CAD build for the part. Positions are in the model's coordinates, mm. Face numbers are marked on the shaded views. A direction names the side the tool comes from. Give positions to 0.01 mm unless a question says otherwise; leave off trailing zeros. Write each loop counter-clockwise with the first axis right and the second up, starting at its lowest first coordinate (ties: lowest second). Pieces come first, ordered by that corner, then holes. Notation, with made-up numbers: (25, 58) - (55, 58) arc R25 ccw to (55, 70) - close; hole circle Ø1 at (56.25, 43.25). An arc over 180 degrees is marked (long way). Answer as a JSON object with one key per item and string values.
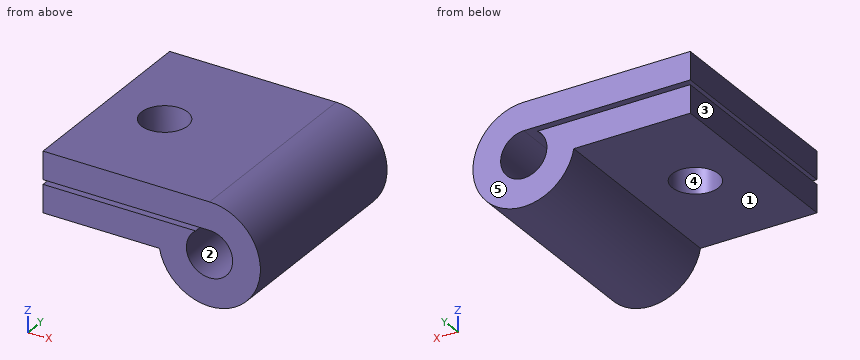
from build123d import *

# Parameters (mm, degrees)
SALIENTE_EXTRUIR1_DEPTH = 22
CROQUIS2_R              = 2.5
CORTAR_EXTRUIR1_DEPTH   = 15


with BuildPart() as part:
    # Croquis1 → Saliente-Extruir1 (new body)
    with BuildSketch(Plane(origin=(0, 0, 0), x_dir=(1, 0, 0), z_dir=(0, 1, 0))):
        with BuildLine():
            Line((0, -5.5), (-18, -5.5))
            Line((-18, -5.5), (-18, -2.5))
            Line((-18, -2.5), (-7.399590065, -2.5))
            Line((-7.399590065, -2.5), (0, -2.5))
            ThreePointArc((0, -2.5), (0.790569415, 2.371708245), (-1.5, -2))
            Line((-1.5, -2), (-6.46658194, -2))
            Line((-6.46658194, -2), (-18, -2))
            Line((-18, -2), (-18, 1))
            Line((-18, 1), (-5.408326913, 1))
            ThreePointArc((-5.408326913, 1), (4.227883631, 3.51781182), (0, -5.5))
        make_face()
    extrude(amount=SALIENTE_EXTRUIR1_DEPTH)

    # Croquis2 → Cortar-Extruir1 (cut)
    with BuildSketch(Plane(origin=(0, 0, -1), x_dir=(-1, 0, 0), z_dir=(0, 0, -1))):
        with Locations((11.704163457, 11)):
            Circle(CROQUIS2_R)
    extrude(amount=-CORTAR_EXTRUIR1_DEPTH, mode=Mode.SUBTRACT)


solid = part.part
Item 1: Cut at D-D (x = -11.5). Give the cut face in (y, z).
Entries:
{"outline": "(0, -1) - (8.51, -1) - (8.51, 2) - (0, 2) - close; (0, 2.5) - (8.51, 2.5) - (8.51, 5.5) - (0, 5.5) - close; (13.49, -1) - (22, -1) - (22, 2) - (13.49, 2) - close; (13.49, 2.5) - (22, 2.5) - (22, 5.5) - (13.49, 5.5) - close"}
Item 2: Cut at B-B (y = 11). Give the cut face in (x, z), and give its area (3 significant figures).
Entries:
{"outline": "(-18, -1) - (-14.2, -1) - (-14.2, 2) - (-18, 2) - close; (-18, 2.5) - (-14.2, 2.5) - (-14.2, 5.5) - (-18, 5.5) - close; (-9.2, -1) - (-5.41, -1) arc R5.5 ccw (long way) to (0, 5.5) - (-9.2, 5.5) - (-9.2, 2.5) - (0, 2.5) arc R2.5 cw (long way) to (-1.5, 2) - (-9.2, 2) - close", "area": "125 mm2"}
Item 3: Cut at C-C (x = -4). Give the cut face in (y, z), and give its area (3 significant figures).
Entries:
{"outline": "(0, -3.77) - (22, -3.77) - (22, 2) - (0, 2) - close; (0, 2.5) - (22, 2.5) - (22, 5.5) - (0, 5.5) - close", "area": "193 mm2"}
Item 4: Which spindle directions (+Z, -Z, +X, -X, +Y, -Y) get a long thin tool onto all of the face, cutting with end or side? Do the marked faces 1 and 2. Say none if no direction does.
Entries:
{"face 1": "-Z, -X, +Y, -Y", "face 2": "+Y, -Y"}
Item 5: Mould opens along Y. For the marked faces 3, 4 and 5 say: +Y half, -Y half, draft (parallel to the pull), parting line (faces both ways), or undercut.
Entries:
{"face 3": "draft", "face 4": "undercut", "face 5": "+Y half"}
Item 6: Probe line 1 (Z direction, x = -11.25, y = 20); line 2 (Z direction, x = -2.25, y = 18); line 3 (X direction, y = 7.75, z = 0). List the from-to ranges inside material, lowest first. Write a range as from..to.
Entries:
{"line 1": "-1..2, 2.5..5.5", "line 2": "-5.02..-1.09, 1.09..2, 2.5..5.5", "line 3": "-18..-2.5, 2.5..5.5"}
Item 7: Cut at A-A (z = 0). Give the cut face in (x, y), and give its area (3 significant figures).
Entries:
{"outline": "(-18, 0) - (-2.5, 0) - (-2.5, 22) - (-18, 22) - close; (2.5, 0) - (5.5, 0) - (5.5, 22) - (2.5, 22) - close; hole circle Ø5 at (-11.7, 11)", "area": "387 mm2"}
Item 8: Flat gauge pins, fed straight in: P1, Ø10, axis at x = -13.5, y = 14.5, coming from the -Z side; P2, Ø4, axis at x = -14, z = -4, coming from the +Y side; P3, Ø9, axis at x = -8, y = 10.5, coming from the -Z side. Where does each tip first touch, or does it go through?
Entries:
{"P1": "z = -1", "P2": "through", "P3": "z = -4.24"}
